```python
from build123d import *

# Parameters (mm, degrees)
BOSS_EXTRUDE1_DEPTH = 12.7
SKETCH3_W           = 5.08
SKETCH3_H           = 5.08
CUT_EXTRUDE1_DEPTH  = 6.35
SKETCH2_R           = 1.5875
CUT_EXTRUDE2_DEPTH  = 3.81
CUT_EXTRUDE3_REACH  = 20.502
SKETCH4_R           = 1.7859375


with BuildPart() as part:
    # Sketch1 → Boss-Extrude1 (new body)
    with BuildSketch(Plane.XY):
        Polygon((0, 0), (0, 7.62), (12.7, 7.62), (12.7, 4.445), (6.35, 4.445), (6.35, 0), align=None)
    extrude(amount=BOSS_EXTRUDE1_DEPTH)

    # Mirror1: part across plane


with BuildPart() as part_1:
    add(part.part)
    add(part.part.mirror(Plane(origin=(0, 0, 12.7), x_dir=(0, 0, 1), z_dir=(-1, 0, 0))))

    # Sketch3 → Cut-Extrude1 (cut)
    with BuildSketch(Plane(origin=(0, 7.62, 0), x_dir=(1, 0, 0), z_dir=(0, 1, 0))):
        with Locations((0, -6.35)):
            Rectangle(SKETCH3_W, SKETCH3_H)
    extrude(amount=-CUT_EXTRUDE1_DEPTH, mode=Mode.SUBTRACT)

    # Sketch2 → Cut-Extrude2 (cut)
    with BuildSketch(Plane.ZY.offset(6.35)):
        with Locations(Location((6.35, 2.8575, 0), (0, 0, 270))):
            Circle(SKETCH2_R)
    extrude(amount=-CUT_EXTRUDE2_DEPTH, mode=Mode.SUBTRACT)

    # Sketch4 → Cut-Extrude3 (cut, up to next)
    with BuildSketch(Plane.XZ.offset(-4.445), mode=Mode.PRIVATE) as cut_extrude3_sk1:
        with Locations((9.525, 6.35)):
            Circle(SKETCH4_R)
    cut_extrude3_tool1 = extrude(cut_extrude3_sk1.sketch, amount=-CUT_EXTRUDE3_REACH, mode=Mode.PRIVATE) & part_1.part
    # Sketch4 → Cut-Extrude3 (cut, up to next)
    with BuildSketch(Plane.XZ.offset(-4.445), mode=Mode.PRIVATE) as cut_extrude3_sk2:
        with Locations((-9.525, 6.35)):
            Circle(SKETCH4_R)
    cut_extrude3_tool2 = extrude(cut_extrude3_sk2.sketch, amount=-CUT_EXTRUDE3_REACH, mode=Mode.PRIVATE) & part_1.part
    add(cut_extrude3_tool1.solids().sort_by_distance((9.525, 4.445, 6.35))[0], mode=Mode.SUBTRACT)
    add(cut_extrude3_tool2.solids().sort_by_distance((-9.525, 4.445, 6.35))[0], mode=Mode.SUBTRACT)


solid = part_1.part
```
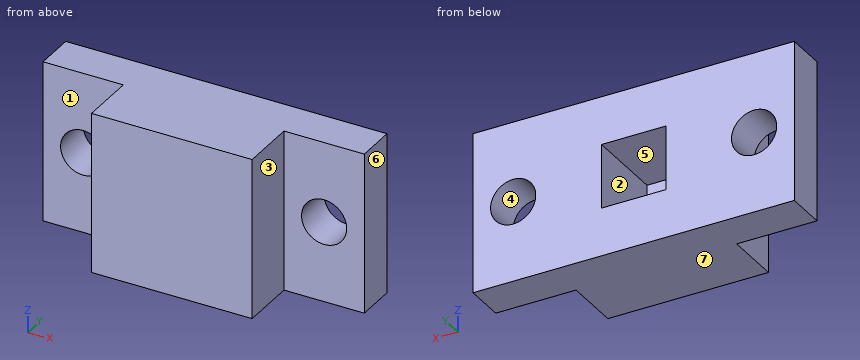
Build history of the part. All positions in model axes, mm. Face numbers are marked on the shaded views. A direction names the side the tool comes from. Give positions to 0.01 mm unless a question says otherwise; leave off trailing zeros. Loops run counter-clockwise (first coordinate to the right, second up) from the corner with the lowest first, then second, coordinate; pieces in that order, holes last.
1) Drop flat-ended pins along their axis: P1, Ø7, axis at x = 10.5, z = 9.5, coming from the -Y side (3 decimals); P2, Ø2, axis at y = 2, z = 7, coming from the +X side; P3, Ø1.5, axis at x = -0.5, y = 4, coming from the -Z side; P4, Ø4, axis at y = 2, z = 4, coming from the -X side. Give the stop position or say it passes through.
Values follow:
P1: stops at y = 4.445
P2: stops at x = 6.35
P3: stops at z = 0
P4: stops at x = -6.35
2) Two-plate mould, pull along X, no slides. Class the marked faces 4, 5, 6 and 7: released by +X, released by -X, zero draft, split by the parting line, or undercut.
Values follow:
face 4: undercut
face 5: undercut
face 6: released by +X
face 7: zero draft
3) Band-saw the part on A-A on z = 5.5. List the corners of the cut face in (x, y) (3 decimals), then the cut area to 3 significant figures.
Values follow:
outline: (-12.7, 4.445) - (-11.096, 4.445) - (-11.096, 7.62) - (-12.7, 7.62) - close; (-7.954, 4.445) - (-6.35, 4.445) - (-6.35, 4.198) - (-2.54, 4.198) - (-2.54, 7.62) - (-7.954, 7.62) - close; (-6.35, 0) - (6.35, 0) - (6.35, 4.445) - (7.954, 4.445) - (7.954, 7.62) - (2.54, 7.62) - (2.54, 1.27) - (-2.54, 1.27) - (-2.54, 1.517) - (-6.35, 1.517) - close; (11.096, 4.445) - (12.7, 4.445) - (12.7, 7.62) - (11.096, 7.62) - close
area: 74.7 mm2
4) Band-saw the part on C-C on y = 4.75. List the corners of the cut face in (x, z) (3 decimals).
Values follow:
outline: (-12.7, 0) - (12.7, 0) - (12.7, 12.7) - (-12.7, 12.7) - close; hole circle Ø3.572 at (-9.525, 6.35); hole (-2.54, 3.81) - (2.54, 3.81) - (2.54, 8.89) - (-2.54, 8.89) - close; hole circle Ø3.572 at (9.525, 6.35)
5) Band-saw the part on B-B on x = -9. List the corners of the cut face in (y, z) (3 decimals).
Values follow:
outline: (4.445, 0) - (7.62, 0) - (7.62, 4.643) - (4.445, 4.643) - close; (4.445, 8.057) - (7.62, 8.057) - (7.62, 12.7) - (4.445, 12.7) - close
6) 3-axis set-ups, long thin cutter, end or side, ignore diameter. For the marked faces 1, 2 and 3: which of +Z, -Z, +X, -X, +Y, -Y reach the whole face in a straight line?
Values follow:
face 1: +Z, -Z, -X, -Y
face 2: +Y
face 3: +Z, -Z, +X, -Y
7) Probe line 1 along Z through (x, y) = (1.5, 6.75); line 2 along X through (y, z) = (7.25, 4.5); line 3 along Y through (x, z) = (8.75, 0.5) (3 decimals). List the from-to ranges inside material, lowest first.
Values follow:
line 1: z = 0 to 3.81, 8.89 to 12.7
line 2: x = -12.7 to -2.54, 2.54 to 12.7
line 3: y = 4.445 to 7.62
8) Band-saw the part on D-D on x = -0.5. List the corners of the cut face in (y, z).
Values follow:
outline: (0, 0) - (7.62, 0) - (7.62, 3.81) - (1.27, 3.81) - (1.27, 8.89) - (7.62, 8.89) - (7.62, 12.7) - (0, 12.7) - close
